```python
from build123d import *

# Parameters (mm, degrees)
SKETCH_1_R          = 2.5
EXTRUDE_1_DEPTH     = 8
SKETCH_2_R          = 0.5
CUT_EXTRUDE_2_DEPTH = 4
SKETCH_3_W          = 1
SKETCH_3_H          = 4
CUT_EXTRUDE_3_DEPTH = 8


with BuildPart() as part:
    # 草图1 → 凸台-拉伸1 (new body)
    with BuildSketch(Plane(origin=(0, 0, 0), x_dir=(0, 0, -1), z_dir=(1, 0, 0))):
        Circle(SKETCH_1_R)
    extrude(amount=EXTRUDE_1_DEPTH)

    # 草图2 → 切除-拉伸2 (cut, symmetric)
    with BuildSketch(Plane(origin=(0, 0, 0), x_dir=(1, 0, 0), z_dir=(0, 1, 0))):
        with Locations(Location((4, 0, 0), (0, 0, 270))):
            Circle(SKETCH_2_R)
    extrude(amount=CUT_EXTRUDE_2_DEPTH, both=True, mode=Mode.SUBTRACT)

    # 草图3 → 切除-拉伸3 (cut)
    with BuildSketch(Plane(origin=(8, 0, 0), x_dir=(0, 0, -1), z_dir=(1, 0, 0))):
        with Locations((0, 2.5)):
            Rectangle(SKETCH_3_W, SKETCH_3_H)
    extrude(amount=-CUT_EXTRUDE_3_DEPTH, mode=Mode.SUBTRACT)


solid = part.part
```
For this review, take the finished solid that the model builds, in its own axes (mm). A direction names the side the tool comes from. Round coordinates to 2 decimals unless told otherwise and drop trailing zeros. Write each loop counter-clockwise with the first axis right and the second up, starting at its lowest first coordinate (ties: lowest second). Pieces come first, ordered by that corner, then holes. Notation, with made-up numbers: (-17, -15.75) -> (17, -15.75) arc R19 cw to (17, 12.25) -> close; hole circle Ø8 at (-27, 19.5). An arc over 180 degrees is marked (long way). Use one line per item in the form item = value.
Q1. Consider section C-C (y = 0). State the section outline as (x, z) points, then the cut area to 3 significant figures.
Resolved:
outline = (0, -2.5) -> (8, -2.5) -> (8, 2.5) -> (0, 2.5) -> close; hole circle Ø1 at (4, 0)
area = 39.2 mm²
Q2. To check wall thickness, follow probe 1 along X at (y, z) = (-0.3, 0); probe 2 along Z at (x, y) = (4, -0.05); probe 3 along Z at (x, y) = (1.75, 0.9). State the ranges of each line that lie inside material, in increasing order. Write a range as from..to.
Resolved:
probe_1 = 0..3.5, 4.5..8
probe_2 = -2.5..-0.5, 0.5..2.5
probe_3 = -2.33..-0.5, 0.5..2.33
Q3. Consider section A-A (z = 0). State the section outline as (x, y) points, then the cut area to 3 significant figures.
Resolved:
outline = (0, -2.5) -> (3.5, -2.5) -> (3.5, 0.5) -> (0, 0.5) -> close; (4.5, -2.5) -> (8, -2.5) -> (8, 0.5) -> (4.5, 0.5) -> close
area = 21.0 mm²
Q4. Consider section D-D (x = 5.75). State the section outline as (y, z) points.
Resolved:
outline = (0.5, -0.5) -> (0.5, 0.5) -> (2.45, 0.5) arc R2.5 ccw (long way) to (2.45, -0.5) -> close
Q5. Clearance check with flat-ended pins moving along their axes: pin 1 Ø2 at (x, y) = (6, 2) entering from +Z; pin 2 Ø0.5 at (x, z) = (6.5, 0) entering from +Y; pin 3 Ø2 at (x, y) = (2.5, 1.5) entering from -Z. State where each tip first meets the part, or that it passes through.
Resolved:
pin_1 = 2.29
pin_2 = 0.5
pin_3 = -2.45
Q6. Consider section B-B (y = 1.35). State the section outline as (x, z) points.
Resolved:
outline = (0, -2.1) -> (8, -2.1) -> (8, -0.5) -> (0, -0.5) -> close; (0, 0.5) -> (8, 0.5) -> (8, 2.1) -> (0, 2.1) -> close
Q7. Machinability: for faces 1 (the flat face through (0, 0, 0)), 2 (the flat face through (4, 1, -0.5)), which of the approach directions +Z, -Z, +X, -X, +Y, -Y give a long, thin tool a straight path to every point of the face, cutting with its end or side? Answer none if there is none.
Resolved:
face_1 = +Z, -Z, -X, +Y, -Y
face_2 = +X, -X, +Y
Q8. The part is to be moulded in two halves that separate along Z. For faces 3 (the cylindrical face through (3.944, -2.046, -1.437)), 4 (the flat face through (8, 0, 0)), 5 (the flat face through (4, 1, 0.5)), say which applies: released by +Z, released by -Z, zero draft, split by the parting line, or undercut.
Resolved:
face_3 = split by the parting line
face_4 = zero draft
face_5 = undercut
